```python
from build123d import *

# Parameters (mm, degrees)
BOSS_EXTRUDE1_DEPTH = 10
SKETCH2_R           = 3
CUT_EXTRUDE1_DEPTH  = 8


with BuildPart() as part:
    # Sketch1 → Boss-Extrude1 (new body)
    with BuildSketch(Plane(origin=(0, 0, 0), x_dir=(1, 0, 0), z_dir=(0, 1, 0))):
        with BuildLine():
            Line((-14.70271565, -10.052675371), (-29.165444207, -10.052675371))
            Line((-29.165444207, -10.052675371), (-29.165444207, -7.552675371))
            Line((-29.165444207, -7.552675371), (-19.04460375, -7.552675371))
            ThreePointArc((-19.04460375, -7.552675371), (-17.652378747, -7.021091902), (-16.731881464, -5.849103764))
            ThreePointArc((-16.731881464, -5.849103764), (1.79728435, 8.947324629), (20.326450163, -5.849103764))
            ThreePointArc((20.326450163, -5.849103764), (21.246947447, -7.021091902), (22.63917245, -7.552675371))
            Line((22.63917245, -7.552675371), (32.849946683, -7.552675371))
            Line((32.849946683, -7.552675371), (32.849946683, -10.052675371))
            Line((32.849946683, -10.052675371), (18.29728435, -10.052675371))
            ThreePointArc((18.29728435, -10.052675371), (1.79728435, 6.447324629), (-14.70271565, -10.052675371))
        make_face()
    extrude(amount=BOSS_EXTRUDE1_DEPTH)

    # Sketch2 → Cut-Extrude1 (cut)
    with BuildSketch(Plane(origin=(0, 0, 7.552675371), x_dir=(-1, 0, 0), z_dir=(0, 0, -1))):
        with Locations((24.165444207, 5)):
            Circle(SKETCH2_R)
        with Locations((-27.849946683, 5)):
            Circle(SKETCH2_R)
    extrude(amount=-CUT_EXTRUDE1_DEPTH, mode=Mode.SUBTRACT)


solid = part.part
```
Here's how the part is built. I have some questions about the finished solid (model axes, mm). A direction names the side the tool comes from. Coordinates: 2 decimals unless noted, no trailing zeros. Loops run counter-clockwise (first coordinate to the right, second up) from the corner with the lowest first, then second, coordinate; pieces in that order, holes last. Notation, with made-up numbers: (23.5, 2.5) - (66.5, 2.5) arc R7 ccw to (66.5, 15.5) - close; hole circle Ø8 at (-6, 65). An arc over 180 degrees is marked (long way). Answer as CSV lines item,"result".
Q1. If we section it at B-B, the plane z = -3: Write out the boundary of the cut face in (x, y), and give its area (3 significant figures).
Response:
outline,"(-12.01, 0) - (-8.3, 0) - (-8.3, 10) - (-12.01, 10) - close; (11.89, 0) - (15.6, 0) - (15.6, 10) - (11.89, 10) - close"
area,"74.3 mm2"
Q2. If I drill on L1, parallel to X at y = 3.25, z = 7.75; L2, parallel to Z at x = -26, y = 9.25; L3, parallel to X at y = 4.5, z = 4.5, over which ranges is the centre line in solid material (lowest first)? Write a range as [from, to].
Response:
L1,"[-29.17, -26.6], [-21.73, -14.54], [18.14, 25.41], [30.29, 32.85]"
L2,"[7.55, 10.05]"
L3,"[-16.37, -13.74], [17.33, 19.97]"
Q3. If we section it at A-A, the plane y = 5: Write out the boundary of the cut face in (x, z), and give its area (3 significant figures).
Response:
outline,"(-29.17, 7.55) - (-27.17, 7.55) - (-27.17, 10.05) - (-29.17, 10.05) - close; (-21.17, 7.55) - (-19.04, 7.55) arc R2.79 cw to (-16.73, 5.85) arc R19 ccw to (20.33, 5.85) arc R2.79 cw to (22.64, 7.55) - (24.85, 7.55) - (24.85, 10.05) - (18.3, 10.05) arc R16.5 cw to (-14.7, 10.05) - (-21.17, 10.05) - close; (30.85, 7.55) - (32.85, 7.55) - (32.85, 10.05) - (30.85, 10.05) - close"
area,"172 mm2"
Q4. If we section it at C-C, the plane x = -22.5: Write out the boundary of the cut face in (y, z).
Response:
outline,"(0, 7.55) - (2.5, 7.55) - (2.5, 10.05) - (0, 10.05) - close; (7.5, 7.55) - (10, 7.55) - (10, 10.05) - (7.5, 10.05) - close"
Q5. If we section it at D-D, the plane x = 21.5: Write out the boundary of the cut face in (y, z).
Response:
outline,"(0, 7.19) - (10, 7.19) - (10, 10.05) - (0, 10.05) - close"
Q6. For pin 1 (3.5 mm diameter, centred on x = -24.17, y = 5, fed in from +Z); pin 2 (8 mm diameter, centred on x = -22.5, z = 4.5, fed in from -Y), each with a flat end and sliding along its axis, tell me the tip position at first contact or that it passes through.
Response:
pin 1,"through"
pin 2,"y = 0"
Q7. We'd pull the mould along Y, two halves only. Please class faces 3 (the face through (-26.937, 3.851, 8.785)), 4 (the face through (2, 10, -7)), 5 (the face through (-26.4, 2.7, 7.553)), 6 (the face through (25.08, 3.85, 8.79)): pulls with the +Y half, pulls with the -Y half, needs draft (parallel to the pull), parting line crosses it, or undercut.
Response:
face 3,"undercut"
face 4,"pulls with the +Y half"
face 5,"needs draft"
face 6,"undercut"
Q8. For faces 1 (the face through (-17.669, 4.93, 7.034)), 2 (the face through (25, 3, 7.553)), which set-ups out of +Z, -Z, +X, -X, +Y, -Y let a thin tool reach every point of the face, with its end or its side?
Response:
face 1,"-Z, -X, +Y, -Y"
face 2,"-Z, +X, +Y, -Y"
